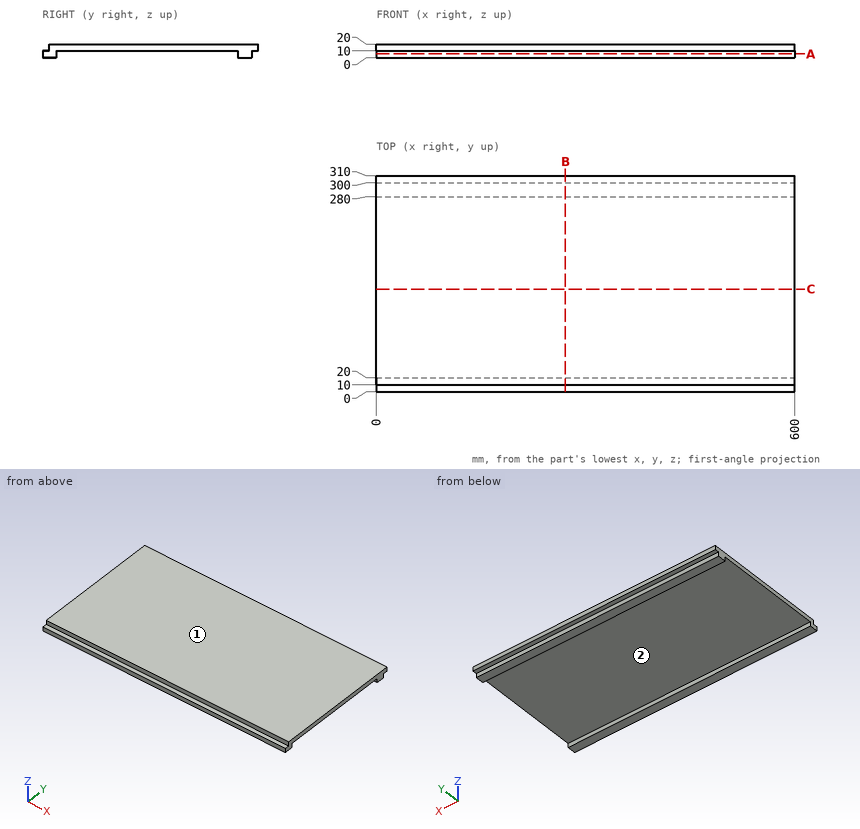
Answer from the drawing. Dimensions are ordinates in mm from the lowest x, y and z of the part. Coordinates: 2 decimals unless noted, no trailing zeros. Loops run counter-clockwise (first coordinate to the right, second up) from the corner with the lowest first, then second, coordinate; pieces in that order, holes last.
1) Section B-B (x = 271) is taken. Give the vertices of the cut face in (y, z).
Results:
outline: (0, 0) - (20, 0) - (20, 10) - (280, 10) - (280, 0) - (300, 0) - (300, 10) - (310, 10) - (310, 20) - (10, 20) - (10, 10) - (0, 10) - close
2) Consider probe 1 along Y at (x, z) = (436.5, 6); probe 2 along Y at (x, z) = (437.5, 18.75); probe 3 along Z at (x, y) = (219, 22). Determine where each line is inside the solid, lowest interval first.
Results:
probe 1: y = 0 to 20, 280 to 300
probe 2: y = 10 to 310
probe 3: z = 10 to 20
3) Section A-A (z = 5.75) is taken. Give the vertices of the cut face in (x, y).
Results:
outline: (0, 0) - (600, 0) - (600, 20) - (0, 20) - close; (0, 280) - (600, 280) - (600, 300) - (0, 300) - close
4) Flat-ended cylindrical pins translate along their axes: pin 1 (11 mm diameter, centred on x = 255.5, z = 7, fed in from +Y); pin 2 (1.5 mm diameter, centred on x = 100, y = 141, fed in from -Z); pin 3 (1 mm diameter, centred on x = 437.5, z = 5.5, fed in from +Y); pin 4 (3 mm diameter, centred on x = 327, y = 2.5, fed in from +Z). Find the tip coordinate at first contact, or state that the pin passes through.
Results:
pin 1: stops at y = 310
pin 2: stops at z = 10
pin 3: stops at y = 300
pin 4: stops at z = 10
5) Section C-C (y = 147.5) is taken. Give the vertices of the cut face in (x, z), plus the area to 3 significant figures.
Results:
outline: (0, 10) - (600, 10) - (600, 20) - (0, 20) - close
area: 6,000 mm2
6) For a pull along Y with two mould halves and no side action, classify the marked faces 1 and 2 as +Y half, -Y half, draft (parallel to the pull), parting line (faces both ways), or undercut.
Results:
face 1: draft
face 2: undercut
